For this review, take the finished solid that the model builds, in its own axes (mm). A direction names the side the tool comes from. Round coordinates to 2 decimals unless told otherwise and drop trailing zeros. Loops run counter-clockwise (first coordinate to the right, second up) from the corner with the lowest first, then second, coordinate; pieces in that order, holes last.
1. To check wall thickness, follow line 1 along Z through (x, y) = (-73.75, 18.5); line 2 along Y through (x, z) = (-81.5, -27.5); line 3 along X through (y, z) = (-9, -20). State the ranges of each line that lie inside material, in increasing order.
2. Tool access review of faces 1 (the flat face through (-81, 37, -23)), 2 (the flat face through (-71, 0, 0)): name each direction out of +Z, -Z, +X, -X, +Y, -Y from which nothing blocks a thin tool from reaching the whole face with its end or side.
3. Clearance check with flat-ended pins moving along their axes: pin 1 Ø6 at (y, z) = (10.5, 27) entering from -X; pin 2 Ø1 at (x, y) = (-76, 8) entering from +Z; pin 3 Ø5 at (x, y) = (-81.5, -27) entering from -Z. State where each tip first meets the part, or that it passes through.
4. Consider section A-A on x = -79.25. State the section outline as (y, z) points, then the cut area to 3 significant figures.
Autodesk Inventor part; units mm, degrees
ref_plane "Work Plane5" through (-81, 0, 0) normal (1, 0, 0) x (0, 1, 0)
ref_plane "XZ Plane" through (0, 0, 0) normal (0, 1, 0) x (-1, 0, 0)
ref_plane "XY Plane" through (0, 0, 0) normal (0, 0, 1) x (1, 0, 0)
ref_plane "Work Plane5" through (-81, 0, 0) normal (1, 0, 0) x (0, 1, 0)
sketch "Sketch9" plane through (-81, 0, 0) normal (1, 0, 0) x (0, 1, 0)
  circle A0 centre (0, 0) radius 36.225
  dimension "d79" = 72.45
extrude "Extrusion5" add sketch "Sketch9" along normal blind 10 draft -8
sketch "Sketch10" plane through (-81, 0, 0) normal (-1, 0, 0) x (0, 0, 1)
  circle A0 centre (0, 0) radius 43.5874
extrude "Extrusion6" add sketch "Sketch10" along normal blind 1
fillet "Fillet12" radius 8 1 edges at (-81, -36.225, 0)
draft "FaceDraft1" angle 45 pull direction (-1, 0, 0) faces at (-81.6667, -40.4135, -16.3281) fixed edges at (-82, 0, -43.5874)
sketch "Sketch16" plane through (0, 0, 0) normal (0, 1, 0) x (-1, 0, 0)
  line L0 (82, -43.5874) -> (82, 43.5874)
  line L1 (82, -43.5874) -> (83.9506, -32.6257) construction
  line L2 (83.9506, -32.6257) -> (84.4455, -26.8642) construction
  line L3 (84.4455, -26.8642) -> (85.3944, -15.8156) construction
  line L4 (85.3944, -15.8156) -> (85.3944, -9.2357) construction
  line L5 (85.3944, -9.2357) -> (84.8986, -0.5811) construction
  line L6 (84.8986, -0.5811) -> (84.8986, 0) construction
  spline S0 degree 4 poles (82, -43.5874) (83.9506, -32.6257) (84.4455, -26.8642) (85.3944, -15.8156) (85.3944, -9.2357) (84.8986, -0.5811) (84.8986, 0) knots 1 1 1 1 1 2 3 4 4 4 4 4
  line L7 (84.8986, 0) -> (82, 0)
  point P0 (0, 0)
revolve "Revolution3" add sketch "Sketch16" angle 360 about axis through (-84.8986, 0, 0) along (1, 0, 0)
ref_plane "Work Plane7" through (-96.5, 0, 0) normal (1, 0, 0) x (0, 0, -1)
sketch "Sketch23" plane through (-96.5, 0, 0) normal (1, 0, 0) x (0, 0, -1)
  line L0 (-47.6775, 46.8192) -> (46.7277, 46.8192) construction
  line L1 (46.7277, 46.8192) -> (46.7277, -47.7154) construction
  line L2 (46.7277, -47.7154) -> (-47.6775, -47.7154) construction
  line L3 (-47.6775, -47.7154) -> (-47.6775, 46.8192) construction
  point P0 (0, 0)
properties part number "BMW Cap dish decal ready to attach" material "Brass, Soft Yellow"
Resolved:
1. line 1: z = -29.95 to 29.95
1. line 2: y = -34.46 to 34.46
1. line 3: x = -84.82 to -71
2. face 1: +X
2. face 2: +Z, -Z, +X, +Y, -Y
3. pin 1: stops at x = -84.51
3. pin 2: stops at z = 35.11
3. pin 3: stops at z = -37.22
4. outline: circle Ø76.37 at (0, 0)
4. area: 4,580 mm2
